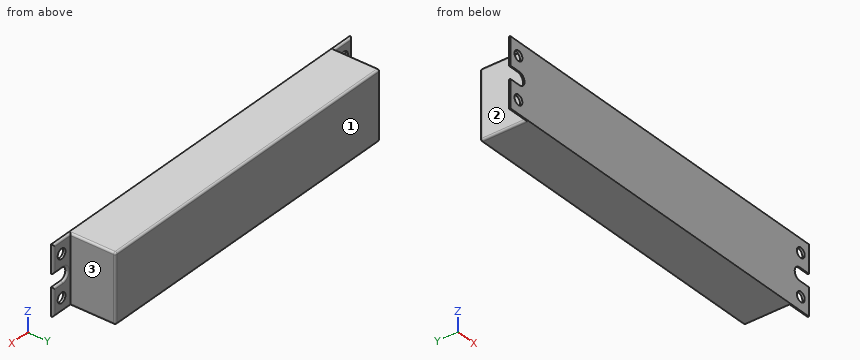
from build123d import *

# Parameters (mm, degrees)
SKETCH1_W                   = 241.3
SKETCH1_H                   = 43.688
BOSS_EXTRUDE1_DEPTH         = 1.524
F_1_4_0_25_DIAMETER_HOLE1_D = 6.35
CUT_EXTRUDE1_DEPTH          = 2.524
SKETCH5_W                   = 213.614
SKETCH5_H                   = 43.688
BOSS_EXTRUDE2_DEPTH         = 28.956
FILLET2_R                   = 1.27


with BuildPart() as part:
    # Sketch1 → Boss-Extrude1 (new body)
    with BuildSketch(Plane(origin=(0, 0, 0), x_dir=(1, 0, 0), z_dir=(0, 1, 0))):
        Rectangle(SKETCH1_W, SKETCH1_H)
    extrude(amount=BOSS_EXTRUDE1_DEPTH)

    # 1/4 (0.25) Diameter Hole1 (through all)
    with Locations(Plane(origin=(0, 1.524, 0), x_dir=(1, 0, 0), z_dir=(0, 1, 0))):
        with Locations((114.046, -13.335), (-114.046, 13.335), (-114.046, -13.335), (114.046, 13.335)):
            Hole(F_1_4_0_25_DIAMETER_HOLE1_D / 2)

    # Sketch4 → Cut-Extrude1 (cut, through all)
    with BuildSketch(Plane(origin=(0, 1.524, 0), x_dir=(1, 0, 0), z_dir=(0, 1, 0))):
        with BuildLine():
            Line((-120.65, 4.064), (-113.2205, 4.064))
            ThreePointArc((-113.2205, 4.064), (-109.1565, 0), (-113.2205, -4.064))
            Line((-113.2205, -4.064), (-120.65, -4.064))
            Line((-120.65, -4.064), (-120.65, 4.064))
        make_face()
        with BuildLine():
            Line((113.2205, 4.064), (120.65, 4.064))
            Line((120.65, 4.064), (120.65, -4.064))
            Line((120.65, -4.064), (113.2205, -4.064))
            ThreePointArc((113.2205, -4.064), (109.1565, 0), (113.2205, 4.064))
        make_face()
    extrude(amount=-CUT_EXTRUDE1_DEPTH, mode=Mode.SUBTRACT)

    # Sketch5 → Boss-Extrude2 (add)
    with BuildSketch(Plane(origin=(0, 1.524, 0), x_dir=(1, 0, 0), z_dir=(0, 1, 0))):
        Rectangle(SKETCH5_W, SKETCH5_H)
    extrude(amount=BOSS_EXTRUDE2_DEPTH)

    # Fillet2
    fillet2_edges = [part.edges().sort_by_distance(p)[0] for p in [
        (-120.65, 1.524, -12.954),
        (-113.7285, 1.524, 21.844),
        (120.65, 1.524, -12.954),
        (120.65, 1.524, 12.954),
        (116.93525, 1.524, -4.064),
        (109.1565, 1.524, 0),
        (116.93525, 1.524, 4.064),
        (-120.65, 1.524, 12.954),
        (-109.1565, 1.524, 0),
        (-116.93525, 1.524, -4.064),
        (-116.93525, 1.524, 4.064),
        (113.7285, 1.524, 21.844),
        (-113.7285, 1.524, -21.844),
        (106.807, 16.002, 21.844),
        (106.807, 16.002, -21.844),
        (-106.807, 16.002, -21.844),
        (-106.807, 16.002, 21.844),
        (106.807, 30.48, 0),
        (113.7285, 1.524, -21.844),
        (0, 30.48, -21.844),
        (-106.807, 30.48, 0),
        (0, 30.48, 21.844),
    ]]
    fillet(fillet2_edges, radius=FILLET2_R)


solid = part.part
Input: part model. Units: mm. Frame: model coordinates. Face numbers are marked on the shaded views. Coordinates: 2 decimals unless noted, no trailing zeros. Order: outer loops, then holes, each group sorted by start corner. A loop starts at its lowest first (then second) coordinate and runs counter-clockwise, first axis right, second up. Notation, with made-up numbers: M -6.5,11.5 L 17.5,11.5 A20 ccw 17.5,16.5 Z; hole C -16.5,17 d3. An arc over 180 degrees is marked long. Answer in a Markdown table with one row per item.
(1) Section query A-A, the plane z = 8. Output: boundary loops of the cut face in (x, y), plus the area to 3 significant figures.
Numbers:
| item | result |
|---|---|
| outline | M -120.65,0 L 120.65,0 L 120.65,0.25 A1.27 ccw 119.38,1.52 L 106.81,1.52 L 106.81,29.21 A1.27 ccw 105.54,30.48 L -105.54,30.48 A1.27 ccw -106.81,29.21 L -106.81,1.52 L -119.38,1.52 A1.27 ccw -120.65,0.25 Z |
| area | 6,550 mm^2 |
(2) Draft query along X for the marked faces 1, 2 and 3. Return one class per face: pulls with the +X half, pulls with the -X half, needs draft (parallel to the pull), parting line crosses it, or undercut.
Numbers:
| item | result |
|---|---|
| face 1 | needs draft |
| face 2 | pulls with the -X half |
| face 3 | pulls with the +X half |
(3) Material intervals for line 1 (X direction, y = 1, z = 13); line 2 (X direction, y = 15.5, z = 5.5); line 3 (Z direction, x = -18.5, y = 29.5), sorted ascending. Write a range as [from, to].
Numbers:
| item | result |
|---|---|
| line 1 | x = [-120.41, -117.2], [-110.89, 110.89], [117.2, 120.41] |
| line 2 | x = [-106.81, 106.81] |
| line 3 | z = [-21.81, 21.81] |
(4) Section query B-B, the plane y = 12. Output: boundary loops of the cut face in (x, z), plus the area to 3 significant figures.
Numbers:
| item | result |
|---|---|
| outline | M -106.81,-20.57 A1.27 ccw -105.54,-21.84 L 105.54,-21.84 A1.27 ccw 106.81,-20.57 L 106.81,20.57 A1.27 ccw 105.54,21.84 L -105.54,21.84 A1.27 ccw -106.81,20.57 Z |
| area | 9,330 mm^2 |
(5) Contact query for flat-ended pins moving along their axis: pin 1 Ø10 at (x, z) = (-115, 3.5) entering from +Y; pin 2 Ø4 at (y, z) = (16.5, -2.5) entering from +X; pin 3 Ø5 at (x, z) = (-114.046, 13.335) entering from +Y; pin 4 Ø4 at (y, z) = (26, 12) entering from -X. Output: stop coordinate, or through.
Numbers:
| item | result |
|---|---|
| pin 1 | stops at y = 1.52 |
| pin 2 | stops at x = 106.81 |
| pin 3 | passes through |
| pin 4 | stops at x = -106.81 |
